CAD build for the part. Positions are in the model's coordinates, mm. Coordinates: 2 decimals unless noted, no trailing zeros. Order: outer loops, then holes, each group sorted by start corner. A loop starts at its lowest first (then second) coordinate and runs counter-clockwise, first axis right, second up. Notation, with made-up numbers: (-1.5, 27.25) - (7.5, 27.25) arc R11 cw to (7.5, 38.25) - close; hole circle Ø4 at (79.25, 43). An arc over 180 degrees is marked (long way). Use one line per item in the form item = value.
```python
from build123d import *

# Parameters (mm, degrees)
F1_DEPTH  = 3
F2_R      = 2
F3_DEPTH  = 13.4
F5_DEPTH  = 15.1
F7_DEPTH  = 28
F9_DEPTH  = 40.9
F10_R     = 2.5
F11_DEPTH = 30.3
F12_DEPTH = 32.7


with BuildPart() as f1:
    # F0 (on Top) → F1 (new body)
    with BuildSketch(Plane.XY):
        with BuildLine():
            Line((0, 0), (51.43121, 70.788987))
            ThreePointArc((51.43121, 70.788987), (0, 87.5), (-51.43121, 70.788987))
            Line((-51.43121, 70.788987), (0, 0))
        make_face()
    extrude(amount=F1_DEPTH)

    # F2 (on Top) → F3 (cut)
    with BuildSketch(Plane.XY):
        with Locations((-38.219705, 52.576175)):
            Circle(F2_R)
    extrude(amount=F3_DEPTH, mode=Mode.SUBTRACT)

    # F4 (on Top) → F5 (cut)
    with BuildSketch(Plane.XY):
        with BuildLine():
            ThreePointArc((0, 42.5), (3.535534, 43.964466), (5, 47.5))
            ThreePointArc((5, 47.5), (-3.535534, 51.035534), (0, 42.5))
        make_face()
    extrude(amount=F5_DEPTH, mode=Mode.SUBTRACT)

    # F6 (on Top) → F7 (cut)
    with BuildSketch(Plane.XY):
        with BuildLine():
            add(Edge.make_bspline(
                [(-32.372009, 44.262763), (-27.721515, 48.913255), (-16.280954, 43.176574), (-9.652664, 43.336935)],
                knots=[0, 0, 0, 0, 22.738201, 22.738201, 22.738201, 22.738201], degree=3))
            Line((-32.372009, 44.262763), (0, 0))
            Line((0, 0), (32.459896, 43.336935))
            add(Edge.make_bspline(
                [(10.232204, 43.336935), (7.958638, 43.336935), (28.130125, 49.419351), (32.459896, 43.336935)],
                knots=[0, 0, 0, 0, 22.227692, 22.227692, 22.227692, 22.227692], degree=3))
            add(Edge.make_bspline(
                [(10.232204, 38.267672), (11.534555, 37.32701), (8.94931, 41.252229), (10.232204, 43.336935)],
                knots=[0, 0, 0, 0, 5.069263, 5.069263, 5.069263, 5.069263], degree=3))
            add(Edge.make_bspline(
                [(-9.652664, 38.267672), (-1.960609, 39.786551), (4.604817, 40.60315), (10.232204, 38.267672)],
                knots=[0, 0, 0, 0, 19.884868, 19.884868, 19.884868, 19.884868], degree=3))
            add(Edge.make_bspline(
                [(-9.652664, 43.336935), (-7.098308, 42.695489), (-10.790724, 37.418947), (-9.652664, 38.267672)],
                knots=[0, 0, 0, 0, 5.069263, 5.069263, 5.069263, 5.069263], degree=3))
        make_face()
    extrude(amount=F7_DEPTH, mode=Mode.SUBTRACT)

    # F8 (on Top) → F9 (cut)
    with BuildSketch(Plane.XY):
        with BuildLine():
            add(Edge.make_bspline(
                [(-31.646983, 62.285967), (-34.494214, 59.307128), (-33.847807, 55.272655), (-30.18681, 53.478997)],
                knots=[0, 0, 0, 0, 8.927196, 8.927196, 8.927196, 8.927196], degree=3))
            add(Edge.make_bspline(
                [(-30.18681, 53.478997), (-24.470332, 52.831151), (-18.69169, 52.237308), (-12.975213, 51.589462)],
                knots=[0, 0, 0, 0, 17.315005, 17.315005, 17.315005, 17.315005], degree=3))
            add(Edge.make_bspline(
                [(-12.975213, 51.589462), (-11.106356, 51.730501), (-9.275662, 53.076804), (-8.538607, 54.607607)],
                knots=[0, 0, 0, 0, 5.365881, 5.365881, 5.365881, 5.365881], degree=3))
            add(Edge.make_bspline(
                [(-6.528673, 58.304172), (-7.200886, 56.853276), (-7.715667, 55.865123), (-8.538607, 54.607607)],
                knots=[0, 0, 0, 0, 4.207662, 4.207662, 4.207662, 4.207662], degree=3))
            add(Edge.make_bspline(
                [(-7.48369, 61.318793), (-6.469775, 60.11533), (-6.048826, 59.233338), (-6.528673, 58.304172)],
                knots=[0, 0, 0, 0, 3.162278, 3.162278, 3.162278, 3.162278], degree=3))
            add(Edge.make_bspline(
                [(-12.531957, 68.392515), (-10.830528, 66.036878), (-9.185119, 63.67443), (-7.48369, 61.318793)],
                knots=[0, 0, 0, 0, 8.690371, 8.690371, 8.690371, 8.690371], degree=3))
            add(Edge.make_bspline(
                [(-15.627065, 69.123868), (-14.042395, 69.763878), (-13.65924, 69.634747), (-12.531957, 68.392515)],
                knots=[0, 0, 0, 0, 3.180341, 3.180341, 3.180341, 3.180341], degree=3))
            add(Edge.make_bspline(
                [(-31.646983, 62.285967), (-26.30701, 64.565267), (-20.967037, 66.844568), (-15.627065, 69.123868)],
                knots=[0, 0, 0, 0, 17.418228, 17.418228, 17.418228, 17.418228], degree=3))
        make_face()
    extrude(amount=F9_DEPTH, mode=Mode.SUBTRACT)

    # F10 (on Top) → F11 (cut)
    with BuildSketch(Plane.XY):
        with Locations((0, 67.25)):
            Circle(F10_R)
    extrude(amount=F11_DEPTH, mode=Mode.SUBTRACT)

    # F8 (on Top) → F12 (cut)
    with BuildSketch(Plane.XY):
        with BuildLine():
            add(Edge.make_bspline(
                [(-31.646983, 62.285967), (-34.494214, 59.307128), (-33.847807, 55.272655), (-30.18681, 53.478997)],
                knots=[0, 0, 0, 0, 8.927196, 8.927196, 8.927196, 8.927196], degree=3))
            add(Edge.make_bspline(
                [(-30.18681, 53.478997), (-24.470332, 52.831151), (-18.69169, 52.237308), (-12.975213, 51.589462)],
                knots=[0, 0, 0, 0, 17.315005, 17.315005, 17.315005, 17.315005], degree=3))
            add(Edge.make_bspline(
                [(-12.975213, 51.589462), (-11.106356, 51.730501), (-9.275662, 53.076804), (-8.538607, 54.607607)],
                knots=[0, 0, 0, 0, 5.365881, 5.365881, 5.365881, 5.365881], degree=3))
            add(Edge.make_bspline(
                [(-6.528673, 58.304172), (-7.200886, 56.853276), (-7.715667, 55.865123), (-8.538607, 54.607607)],
                knots=[0, 0, 0, 0, 4.207662, 4.207662, 4.207662, 4.207662], degree=3))
            add(Edge.make_bspline(
                [(-7.48369, 61.318793), (-6.469775, 60.11533), (-6.048826, 59.233338), (-6.528673, 58.304172)],
                knots=[0, 0, 0, 0, 3.162278, 3.162278, 3.162278, 3.162278], degree=3))
            add(Edge.make_bspline(
                [(-12.531957, 68.392515), (-10.830528, 66.036878), (-9.185119, 63.67443), (-7.48369, 61.318793)],
                knots=[0, 0, 0, 0, 8.690371, 8.690371, 8.690371, 8.690371], degree=3))
            add(Edge.make_bspline(
                [(-15.627065, 69.123868), (-14.042395, 69.763878), (-13.65924, 69.634747), (-12.531957, 68.392515)],
                knots=[0, 0, 0, 0, 3.180341, 3.180341, 3.180341, 3.180341], degree=3))
            add(Edge.make_bspline(
                [(-31.646983, 62.285967), (-26.30701, 64.565267), (-20.967037, 66.844568), (-15.627065, 69.123868)],
                knots=[0, 0, 0, 0, 17.418228, 17.418228, 17.418228, 17.418228], degree=3))
        make_face()
    extrude(amount=F12_DEPTH, mode=Mode.SUBTRACT)


solid = f1.part
```
Item 1: Two-plate mould, pull along X, no slides. Class faces 1 (the face through (-34.67, 47.72, 1.48)), 2 (the face through (41.545, 57.181, 1.479)), 3 (the face through (-36.58, 53.72, 1.48)): +X half, -X half, draft (parallel to the pull), parting line (faces both ways), or undercut.
Derived:
face_1 = -X half
face_2 = +X half
face_3 = undercut
Item 2: Drill centre lines: line 1 (Y direction, x = 0, z = 2.4); line 2 (Y direction, x = -0.5, z = 2.45); line 3 (Y direction, x = -20, z = 2.75). Where is each one in solid material? Low to high. Write a range as [from, to].
Derived:
line_1 = [39.66, 42.5], [52.5, 64.75], [69.75, 87.5]
line_2 = [39.63, 42.53], [52.47, 64.8], [69.7, 87.5]
line_3 = [45.12, 52.36], [67.26, 85.18]
Item 3: Cut at A-A, the plane z = 1.55. State how many separate pieces and enclosed holes the cut face has, plus the area to 3 significant figures.
Derived:
separate_pieces = 1
enclosed_holes = 3
area = 3,010 mm²
Item 4: Drop a flat-ended pin along its axis: pin 1 (1 mm diameter, centred on y = 80.5, z = 1.5, fed in from +X). Give the stop position or say it passes through.
Derived:
pin_1 = 35.44
Item 5: Cut at C-C, the plane x = 34. Write the cut outline in (y, z).
Derived:
outline = (46.8, 0) - (80.62, 0) - (80.62, 3) - (46.8, 3) - close
Item 6: Cut at D-D, the plane y = 82. Write the cut outline in (x, z), plus the area to 3 significant figures.
Derived:
outline = (-30.53, 0) - (30.53, 0) - (30.53, 3) - (-30.53, 3) - close
area = 183 mm²
